```python
from build123d import *

# Parameters (mm, degrees)
F0_R     = 11.24966
F2_DEPTH = 6.35
F1_R     = 2.38125
F3_DEPTH = 25.4


with BuildPart() as f2:
    # F0 (on Top) → F2 (new body)
    with BuildSketch(Plane.XY):
        with BuildLine():
            Line((158.75, 19.05), (-57.15, 19.05))
            ThreePointArc((-57.15, 19.05), (-76.2, 0), (-57.15, -19.05))
            Line((-57.15, -19.05), (158.75, -19.05))
            ThreePointArc((158.75, -19.05), (177.8, 0), (158.75, 19.05))
        make_face()
        with Locations((-50.8, 0)):
            Circle(F0_R, mode=Mode.SUBTRACT)
        with Locations((50.8, 0)):
            Circle(F0_R, mode=Mode.SUBTRACT)
        with Locations((152.4, 0)):
            Circle(F0_R, mode=Mode.SUBTRACT)
    extrude(amount=F2_DEPTH)

    # F1 (on face) → F3 (cut)
    with BuildSketch(Plane.XY):
        Circle(F1_R)
        with Locations((101.6, 0)):
            Circle(F1_R)
    extrude(amount=F3_DEPTH, mode=Mode.SUBTRACT)


solid = f2.part
```
Here's how the part is built. I have some questions about the finished solid (model axes, mm). Coordinates: 2 decimals unless noted, no trailing zeros. Order: outer loops, then holes, each group sorted by start corner. A loop starts at its lowest first (then second) coordinate and runs counter-clockwise, first axis right, second up.
1) We'd pull the mould along X, two halves only. Please class faces 1 (the face through (52, 19.05, 3)), 2 (the face through (-76.195, 0.419, 3.131)), 3 (the face through (163.13, 3.38, 3.13)): +X half, -X half, draft (parallel to the pull), parting line (faces both ways), or undercut.
2) Imagine slicing it at B-B on y = 0. List the corners of the cut face in (x, z) for me.
3) Imagine slicing it at A-A on x = 50.8. List the corners of the cut face in (y, z) for me, and give its area (3 significant figures).
4) Will this pin go through, and if not, where does the flat tip stop? pin 1 (20 mm diameter, centred on x = 50.8, y = 0, fed in from -Z).
5) I need wall thicknesses on line 1 (Y direction, x = 0, z = 2.75); line 2 (Y direction, x = 50.8, z = 3.25); line 3 (X direction, y = 4.5, z = 0.75). Which ranges of each line are inside material? Lowest first, please.
6) Imagine slicing it at D-D on x = 0. List the corners of the cut face in (y, z) for me, and give its area (3 significant figures).
7) Imagine slicing it at C-C on z = 4.25. List the corners of the cut face in (x, y) for me.
Response values:
1. face 1: draft
1. face 2: -X half
1. face 3: undercut
2. outline: (-76.2, 0) - (-62.05, 0) - (-62.05, 6.35) - (-76.2, 6.35) - close; (-39.55, 0) - (-2.38, 0) - (-2.38, 6.35) - (-39.55, 6.35) - close; (2.38, 0) - (39.55, 0) - (39.55, 6.35) - (2.38, 6.35) - close; (62.05, 0) - (99.22, 0) - (99.22, 6.35) - (62.05, 6.35) - close; (103.98, 0) - (141.15, 0) - (141.15, 6.35) - (103.98, 6.35) - close; (163.65, 0) - (177.8, 0) - (177.8, 6.35) - (163.65, 6.35) - close
3. outline: (-19.05, 0) - (-11.25, 0) - (-11.25, 6.35) - (-19.05, 6.35) - close; (11.25, 0) - (19.05, 0) - (19.05, 6.35) - (11.25, 6.35) - close
3. area: 99.1 mm2
4. pin 1: passes through
5. line 1: y = -19.05 to -2.38, 2.38 to 19.05
5. line 2: y = -19.05 to -11.25, 11.25 to 19.05
5. line 3: x = -75.66 to -61.11, -40.49 to 40.49, 61.11 to 142.09, 162.71 to 177.26
6. outline: (-19.05, 0) - (-2.38, 0) - (-2.38, 6.35) - (-19.05, 6.35) - close; (2.38, 0) - (19.05, 0) - (19.05, 6.35) - (2.38, 6.35) - close
6. area: 212 mm2
7. outline: (-57.15, -19.05) - (158.75, -19.05) arc R19.05 ccw to (158.75, 19.05) - (-57.15, 19.05) arc R19.05 ccw to start; hole circle Ø22.5 at (-50.8, 0); hole circle Ø4.76 at (0, 0); hole circle Ø22.5 at (50.8, 0); hole circle Ø4.76 at (101.6, 0); hole circle Ø22.5 at (152.4, 0)
